from build123d import *

# Parameters (mm, degrees)
F1_DEPTH = 60
F3_DEPTH = 30.66775
F4_W     = 60
F4_H     = 20
F5_DEPTH = 10
F7_DEPTH = 20.001


with BuildPart() as f1:
    # F0 (on Right) → F1 (new body)
    with BuildSketch(Plane.YZ):
        Polygon((0, 10.099097), (0, 0), (30.66675, 0), (30.66675, 40.234312), (10.576608, 40.234312), (10.576608, 10.099097), align=None)
    extrude(amount=-F1_DEPTH)

    # F2 (on face) → F3 (cut, through all)
    with BuildSketch(Plane(origin=(0, 30.66675, 0), x_dir=(-1, 0, 0), z_dir=(0, 1, 0))):
        with BuildLine():
            Line((50, 40.234312), (10, 40.234312))
            ThreePointArc((10, 40.234312), (30, 20.234312), (50, 40.234312))
        make_face()
    extrude(amount=-F3_DEPTH, mode=Mode.SUBTRACT)

    # F4 (on face) → F5 (join)
    with BuildSketch(Plane.XZ):
        with Locations((-30, 10)):
            Rectangle(F4_W, F4_H)
    extrude(amount=F5_DEPTH)

    # F6 (on face) → F7 (cut, through all)
    with BuildSketch(Plane.XY.offset(20)):
        Polygon((0, 0), (-20, -10), (0, -10), align=None)
        Polygon((-40, -10), (-60, 0), (-60, -10), align=None)
    extrude(amount=-F7_DEPTH, mode=Mode.SUBTRACT)


solid = f1.part
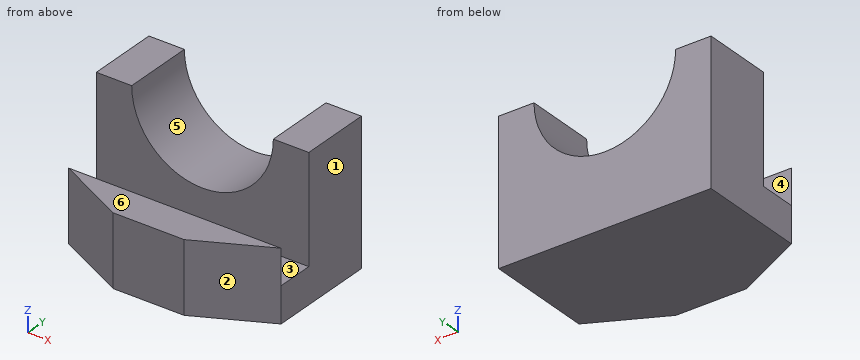
Here's how the part is built. I have some questions about the finished solid (model axes, mm). Face numbers are marked on the shaded views. A direction names the side the tool comes from. Coordinates: 2 decimals unless noted, no trailing zeros. Write each loop counter-clockwise with the first axis right and the second up, starting at its lowest first coordinate (ties: lowest second). Pieces come first, ordered by that corner, then holes.
1) If we section it at A-A (z = 31): List the corners of the cut face in (x, y) for me.
Filled in:
outline: (-60, 10.58) - (-47.74, 10.58) - (-47.74, 30.67) - (-60, 30.67) - close; (-12.26, 10.58) - (0, 10.58) - (0, 30.67) - (-12.26, 30.67) - close
2) If we section it at B-B (x = -51): List the corners of the cut face in (y, z) for me.
Filled in:
outline: (-4.5, 0) - (30.67, 0) - (30.67, 40.23) - (10.58, 40.23) - (10.58, 10.1) - (0, 10.1) - (0, 20) - (-4.5, 20) - close
3) I'm going to push flat-ended pins straight in: pin 1 (5 mm diameter, centred on x = -21, y = -7.5, fed in from +Z); pin 2 (12 mm diameter, centred on x = -26.5, y = 23, fed in from +Z); pin 3 (3 mm diameter, centred on x = -12, y = 3, fed in from +Z). Where does each tip first touch, or does it pass through?
Filled in:
pin 1: stops at z = 20
pin 2: stops at z = 22.63
pin 3: stops at z = 10.1
4) If we section it at D-D (z = 9): List the corners of the cut face in (x, y) for me.
Filled in:
outline: (-60, 0) - (-40, -10) - (-20, -10) - (0, 0) - (0, 30.67) - (-60, 30.67) - close
5) If I drill on line 1 (Y direction, x = -39.5, z = 11); line 2 (Y direction, x = -49, z = 29.5); line 3 (Z direction, x = -13, y = 4), over which ranges is the centre line in solid material (lowest first)?
Filled in:
line 1: y = -10 to 0, 10.58 to 30.67
line 2: y = 10.58 to 30.67
line 3: z = 0 to 10.1
6) Which directions (+Z, -Z, +X, -X, +Y, -Y) give clear straight access to the entire face, cutting with the end or side of a thin tool? Please do the marked faces 4, 5 and 6.
Filled in:
face 4: +Z, +X, -X
face 5: +Z, +Y, -Y
face 6: +Z, +X, -X, -Y
7) If we section it at C-C (y = -3): List the corners of the cut face in (x, z) for me.
Filled in:
outline: (-54, 0) - (-6, 0) - (-6, 20) - (-54, 20) - close
8) Thinking about a two-plate mould opening in Y: for the marked faces 1, 2 and 3, which applies, +Y half, -Y half, draft (parallel to the pull), parting line (faces both ways), or undercut?
Filled in:
face 1: draft
face 2: -Y half
face 3: undercut
